```python
from build123d import *

# Parameters (mm, degrees)
SKETCH_R         = 1.55
PAD_DEPTH        = 5
SKETCH001_R      = 7.5
PAD001_DEPTH     = 8.4
CHAMFER_SIZE     = 1
CHAMFER001_SIZE2 = 3
CHAMFER001_SIZE  = 7


with BuildPart() as part:
    # Sketch → Pad (new body)
    with BuildSketch(Plane.XY):
        Circle(SKETCH_R)
    extrude(amount=-PAD_DEPTH)

    # Sketch001 → Pad001 (join)
    with BuildSketch(Plane.XY):
        Circle(SKETCH001_R)
    extrude(amount=PAD001_DEPTH)

    # Chamfer
    chamfer_edges = [part.edges().sort_by_distance(p)[0] for p in [
        (-1.55, 0, -5),
    ]]
    chamfer(chamfer_edges, length=CHAMFER_SIZE)

    # Chamfer001
    chamfer001_edges = [part.edges().sort_by_distance(p)[0] for p in [
        (-7.5, 0, 8.4),
    ]]
    chamfer001_side = part.faces().sort_by_distance((-7.5, 0, 4.2))[0]
    chamfer(chamfer001_edges, length=CHAMFER001_SIZE, length2=CHAMFER001_SIZE2, reference=chamfer001_side)


solid = part.part
```
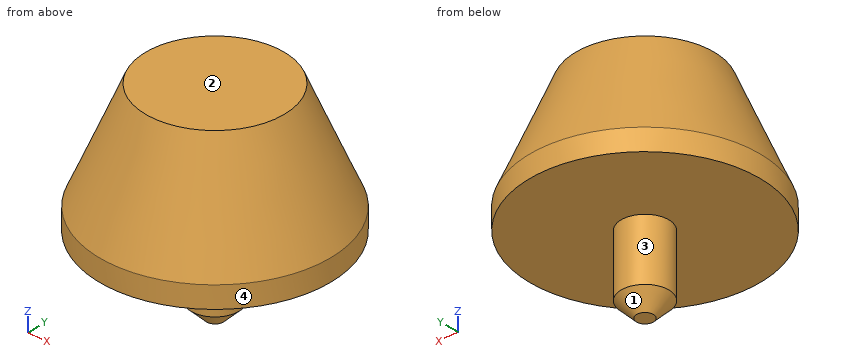
Build history of the part. All positions in model axes, mm. Face numbers are marked on the shaded views. A direction names the side the tool comes from. Round coordinates to 2 decimals unless told otherwise and drop trailing zeros. Write each loop counter-clockwise with the first axis right and the second up, starting at its lowest first coordinate (ties: lowest second). Pieces come first, ordered by that corner, then holes. Notation, with made-up numbers: (83.5, 65) -> (111.5, 65) arc R11 cw to (111.5, 79) -> close; hole circle Ø2 at (-31, -19). An arc over 180 degrees is marked (long way). Put each result on its own line as item: value.
Item 1: Slice it at C-C, the plane z = 0.5. Give the cut face in (x, y).
Here are the results:
outline: circle Ø15 at (0, 0)
Item 2: Flat gauge pins, fed straight in: P1, Ø2, axis at x = -1, z = 5, coming from the -Y side; P2, Ø1.5, axis at y = 5, z = 6.5, coming from the -X side; P3, Ø1, axis at x = 3, y = -6, coming from the +Z side. Where does each tip first touch, or does it go through?
Here are the results:
P1: stops at y = -6.33
P2: stops at x = -3.32
P3: stops at z = 4.41
Item 3: Slice it at A-A, the plane x = 0. Give the cut face in (y, z).
Here are the results:
outline: (-7.5, 0) -> (-1.55, 0) -> (-1.55, -4) -> (-0.55, -5) -> (0.55, -5) -> (1.55, -4) -> (1.55, 0) -> (7.5, 0) -> (7.5, 1.4) -> (4.5, 8.4) -> (-4.5, 8.4) -> (-7.5, 1.4) -> close
Item 4: Tool access for the marked faces 3 and 4: list every direction of +Z, -Z, +X, -X, +Y, -Y with a clear straight run to the whole face (end or side of a thin tool).
Here are the results:
face 3: -Z
face 4: +Z, -Z
Item 5: Two-plate mould, pull along Y, no slides. Class the marked faces 1 and 2: pulls with the +Y half, pulls with the -Y half, needs draft (parallel to the pull), parting line crosses it, or undercut.
Here are the results:
face 1: parting line crosses it
face 2: needs draft
Item 6: Slice it at D-D, the plane z = 2.75. Give the cut face in (x, y).
Here are the results:
outline: circle Ø13.84 at (0, 0)
Item 7: Wall check: probe 1 along Z at (x, y) = (-2, -1.5); probe 2 along Y at (x, z) = (0.25, 4.75); probe 3 along Z at (x, y) = (0.5, 6.25). Give the ranges that are in metal, low to high. Write a range as from..to.
Here are the results:
probe 1: z = 0..8.4
probe 2: y = -6.06..6.06
probe 3: z = 0..4.27
